from build123d import *

# Parameters (mm, degrees)
SKETCH1_W           = 35
SKETCH1_H           = 24
BOSS_EXTRUDE1_DEPTH = 3
CUT_EXTRUDE1_DEPTH  = 7
FILLET1_R           = 4
FILLET2_R           = 0.8


with BuildPart() as part:
    # Sketch1 → Boss-Extrude1 (new body)
    with BuildSketch(Plane(origin=(0, 0, 0), x_dir=(1, 0, 0), z_dir=(0, 1, 0))):
        with Locations((17.5, 12)):
            Rectangle(SKETCH1_W, SKETCH1_H)
    extrude(amount=BOSS_EXTRUDE1_DEPTH)

    # Sketch2 → Cut-Extrude1 (cut)
    with BuildSketch(Plane(origin=(0, 3, 0), x_dir=(1, 0, 0), z_dir=(0, 1, 0))):
        with BuildLine():
            Line((6.6, 19), (6.6, 5))
            ThreePointArc((6.6, 5), (5, 3.4), (3.4, 5))
            Line((3.4, 5), (3.4, 19))
            ThreePointArc((3.4, 19), (5, 20.6), (6.6, 19))
        make_face()
        with BuildLine():
            Line((28.4, 19), (28.4, 5))
            ThreePointArc((28.4, 5), (30, 3.4), (31.6, 5))
            Line((31.6, 5), (31.6, 19))
            ThreePointArc((31.6, 19), (30, 20.6), (28.4, 19))
        make_face()
    extrude(amount=-CUT_EXTRUDE1_DEPTH, mode=Mode.SUBTRACT)

    # Fillet1
    fillet1_edges = [part.edges().sort_by_distance(p)[0] for p in [
        (0, 1.5, 0),
        (0, 1.5, -24),
        (35, 1.5, -24),
        (35, 1.5, 0),
    ]]
    fillet(fillet1_edges, radius=FILLET1_R)

    # Fillet2
    fillet2_edges = [part.edges().sort_by_distance(p)[0] for p in [
        (0, 0, -12),
        (0, 3, -12),
        (17.5, 0, 0),
        (17.5, 0, -24),
        (35, 0, -12),
        (33.828427125, 0, -22.828427125),
        (33.828427125, 0, -1.171572875),
        (1.171572875, 0, -1.171572875),
        (1.171572875, 0, -22.828427125),
        (17.5, 3, -24),
        (17.5, 3, 0),
        (35, 3, -12),
        (33.828427125, 3, -22.828427125),
        (33.828427125, 3, -1.171572875),
        (1.171572875, 3, -1.171572875),
        (1.171572875, 3, -22.828427125),
    ]]
    fillet(fillet2_edges, radius=FILLET2_R)


solid = part.part
CAD build for the part. Positions are in the model's coordinates, mm. A direction names the side the tool comes from. Give positions to 0.01 mm unless a question says otherwise; leave off trailing zeros. Loops run counter-clockwise (first coordinate to the right, second up) from the corner with the lowest first, then second, coordinate; pieces in that order, holes last. Notation, with made-up numbers: M 80,24 L 133,24 A19 ccw 133,39 Z; hole C -10.5,-19 d11. An arc over 180 degrees is marked long. Answer in a Markdown table with one row per item. Add a question column.
Item 1: Tool access for faces 4 (the face through (30, 1.5, -3.4)), 5 (the face through (0, 1, -12)): list every direction of +Z, -Z, +X, -X, +Y, -Y with a clear straight run to the whole face (end or side of a thin tool).
Item 2: Probe probe 1 along X at (y, z) = (1.7, -12.75); probe 2 along X at (y, z) = (0.2, -17.75); probe 3 along Z at (x, y) = (16.5, 0.7). List the from-to ranges inside material, lowest first.
Item 3: Mould opens along X. For faces 1 (the face through (17, 1, -24)), 2 (the face through (5, 1.5, -3.4)), 3 (the face through (35, 1, -12)) say: +X half, -X half, draft (parallel to the pull), parting line (faces both ways), or undercut.
Item 4: Band-saw the part on C-C on x = 30. Give the cut face in (y, z).
Item 5: Band-saw the part on A-A on z = -17. Give the cut face in (x, y).
Item 6: Band-saw the part on B-B on y = 1.55. Give the cut face in (x, z), then the cut area to 3 significant figures.
Reply:
| question | item | result |
|---|---|---|
| 1 | face 4 | +Y, -Y |
| 1 | face 5 | +Z, -Z, -X, +Y, -Y |
| 2 | probe 1 | x = 0 to 3.4, 6.6 to 28.4, 31.6 to 35 |
| 2 | probe 2 | x = 0.27 to 3.4, 6.6 to 28.4, 31.6 to 34.73 |
| 2 | probe 3 | z = -23.99 to -0.01 |
| 3 | face 1 | draft |
| 3 | face 2 | undercut |
| 3 | face 3 | +X half |
| 4 | outline | M 0,-23.2 A0.8 ccw 0.8,-24 L 2.2,-24 A0.8 ccw 3,-23.2 L 3,-20.6 L 0,-20.6 Z; M 0,-3.4 L 3,-3.4 L 3,-0.8 A0.8 ccw 2.2,0 L 0.8,0 A0.8 ccw 0,-0.8 Z |
| 5 | outline | M 0,0.8 A0.8 ccw 0.8,0 L 3.4,0 L 3.4,3 L 0.8,3 A0.8 ccw 0,2.2 Z; M 6.6,0 L 28.4,0 L 28.4,3 L 6.6,3 Z; M 31.6,0 L 34.2,0 A0.8 ccw 35,0.8 L 35,2.2 A0.8 ccw 34.2,3 L 31.6,3 Z |
| 6 | outline | M 0,-20 A4 ccw 4,-24 L 31,-24 A4 ccw 35,-20 L 35,-4 A4 ccw 31,0 L 4,0 A4 ccw 0,-4 Z; hole M 3.4,-19 A1.6 ccw 6.6,-19 L 6.6,-5 A1.6 ccw 3.4,-5 Z; hole M 28.4,-19 A1.6 ccw 31.6,-19 L 31.6,-5 A1.6 ccw 28.4,-5 Z |
| 6 | area | 721 mm^2 |
